from build123d import *

# Parameters (mm, degrees)
BOSS_EXTRUDE1_DEPTH = 5
FILLET2_R           = 5
SKETCH2_W           = 86
SKETCH2_H           = 7.5
SKETCH2_W_2         = 10
SKETCH2_H_2         = 50
CUT_EXTRUDE1_DEPTH  = 161.667358228


with BuildPart() as part:
    # Sketch1 → Boss-Extrude1 (new body)
    with BuildSketch(Plane(origin=(0, 0, 0), x_dir=(1, 0, 0), z_dir=(0, 1, 0))):
        Polygon((-29, -17.5), (-31.5, -17.5), (-31.5, 17.5), (31.5, 17.5), (31.5, -17.5), (29, -17.5), (29, -30), (33, -30), (33, -90), (133, -90), (133, -75), (40, -75), (40, 30), (-20, 30), (-20, 90), (-40, 90), (-40, -30), (-29, -30), align=None)
    extrude(amount=BOSS_EXTRUDE1_DEPTH)

    # Fillet2
    fillet2_edges = [part.edges().sort_by_distance(p)[0] for p in [
        (-40, 2.5, -90),
        (-20, 2.5, -90),
        (40, 2.5, -30),
        (33, 2.5, 90),
        (133, 2.5, 90),
        (133, 2.5, 75),
    ]]
    fillet(fillet2_edges, radius=FILLET2_R)

    # Sketch2 → Cut-Extrude1 (cut, through all)
    with BuildSketch(Plane(origin=(0, 5, 0), x_dir=(1, 0, 0), z_dir=(0, 1, 0))):
        with Locations((83, -82.5)):
            Rectangle(SKETCH2_W, SKETCH2_H)
        with Locations((-30, 60)):
            Rectangle(SKETCH2_W_2, SKETCH2_H_2)
    extrude(amount=-CUT_EXTRUDE1_DEPTH, mode=Mode.SUBTRACT)


solid = part.part
Check sheet for the modelled part. Datum: model origin and axes. Units: mm. A direction names the side the tool comes from. Give positions to 0.01 mm unless a question says otherwise; leave off trailing zeros. Order: outer loops, then holes, each group sorted by start corner. A loop starts at its lowest first (then second) coordinate and runs counter-clockwise, first axis right, second up. Notation, with made-up numbers: M -18.75,-8.75 L 17.25,-8.75 A21 ccw 17.25,17.25 Z; hole C 18,-30.5 d3. An arc over 180 degrees is marked long. Answer as CSV lines item,"result". Start each with the question number.
Item 1: Cross-section at D-D on z = 33.5. Enter the section's corners in (x, y), plus the area to 3 significant figures.
Item 2: Gauge pin test, flat ends, axial feed: P1, Ø2.5, axis at y = 3.5, z = -62, coming from the +X side; P2, Ø2.5, axis at x = -32, y = 2, coming from the +Z side; P3, Ø8, axis at x = 7, z = -36.5, coming from the -Y side; P4, Ø2.5, axis at y = 3.5, z = 21, coming from the +X side. Record the tip position at first contact, or that the pin passes through.
Item 3: Tool access check on faces 1 (the face through (29, 2, 24)), 2 (the face through (-20, 2, -57)), 3 (the face through (-35, 3, -60)), 4 (the face through (34, 3, 88)). Record the directions out of +Z, -Z, +X, -X, +Y, -Y that give a thin tool (end or side, any length) a straight path to the whole face; none if there is none.
Item 4: Thickness scan on line 1 (Z direction, x = 113.5, y = 2.65); line 2 (X direction, y = 2.3, z = -14); line 3 (X direction, y = 3.2, z = -65). Record the ranges inside material, lowest first. Write a range as [from, to].
Item 5: Cross-section at B-B on y = 1.4. State how many separate pieces and enclosed holes the cut face has, plus the area to 3 significant figures.
Item 6: Cross-section at C-C on x = 93. Enter the section's corners in (y, z).
Item 7: Cross-section at A-A on z = -1. Enter the section's corners in (x, y).
Item 8: Mould release check, pull along Z, two halves, no side actions. Record for faces 5 (the face through (132, 3, 77)), 6 (the face through (8, 0, -20)), 7 (the face through (82, 3, 78.75)): +Z half, -Z half, draft (parallel to the pull), parting line (faces both ways), or undercut.
Established:
1,outline,"M 33,0 L 40,0 L 40,5 L 33,5 Z"
1,area,"35.0 mm^2"
2,P1,"stops at x = -20"
2,P2,"stops at z = 30"
2,P3,"passes through"
2,P4,"stops at x = 40"
3,face 1,"+Z, +Y, -Y"
3,face 2,"-Z, +X, +Y, -Y"
3,face 3,"+Y, -Y"
3,face 4,"+Z, -X, +Y, -Y"
4,line 1,"z = [75, 78.75], [86.25, 90]"
4,line 2,"x = [-40, -31.5], [31.5, 40]"
4,line 3,"x = [-40, -35], [-25, -20]"
5,separate pieces,"1"
5,enclosed holes,"2"
5,area,"3,710 mm^2"
6,outline,"M 0,75 L 5,75 L 5,78.75 L 0,78.75 Z; M 0,86.25 L 5,86.25 L 5,90 L 0,90 Z"
7,outline,"M -40,0 L -31.5,0 L -31.5,5 L -40,5 Z; M 31.5,0 L 40,0 L 40,5 L 31.5,5 Z"
8,face 5,"-Z half"
8,face 6,"draft"
8,face 7,"undercut"
